The drawing under review shows one solid part. Ordinate dimensions are in mm from its lowest x, y, z. A direction names the side the tool comes from. Round coordinates to 2 decimals unless told otherwise and drop trailing zeros. Order: outer loops, then holes, each group sorted by start corner. A loop starts at its lowest first (then second) coordinate and runs counter-clockwise, first axis right, second up. Notation, with made-up numbers: M 80.5,75.25 L 111.5,75.25 A15 ccw 111.5,95.25 Z; hole C 84.5,46.25 d3. An arc over 180 degrees is marked long. Answer as a JSON object with one key per item and string values. Group by question number.
1) The part is to be moulded in two halves that separate along X. For the marked faces 1, 2, 3 and 4, say which applies: +X half, -X half, draft (parallel to the pull), parting line (faces both ways), or undercut.
2) Consider section B-B, the plane y = 14.5. Write out the cut boundary in (x, z).
3) For the marked faces 5, 6 and 7, list the 3-axis set-ups (+Z, -Z, +X, -X, +Y, -Y) from which the entire face can be reached by the end or side of a thin tool; tool diameter is ignored.
4) To check wall thickness, follow line 1 (X direction, y = 10.75, z = 70.5); line 2 (X direction, y = 3, z = 18); line 3 (X direction, y = 15.75, z = 56). State the ranges of each line that lie inside material, in increasing order.
5) Consider section C-C, the plane z = 5. Write out the cut boundary in (x, y).
6) Consider section A-A, the plane z = 76. Write out the cut boundary in (x, y), then the cut area to 3 significant figures.
7) Insertion check: pin 1 Ø2.5 at (y, z) = (8, 40.5) entering from +X; pin 2 Ø0.8 at (x, y) = (57, 8) entering from -Z; pin 3 Ø10 at (y, z) = (4.5, 9.5) entering from +X. Each pin has a flat end and moves straight along its axis. Give the tip position at first contact, or say it passes through.
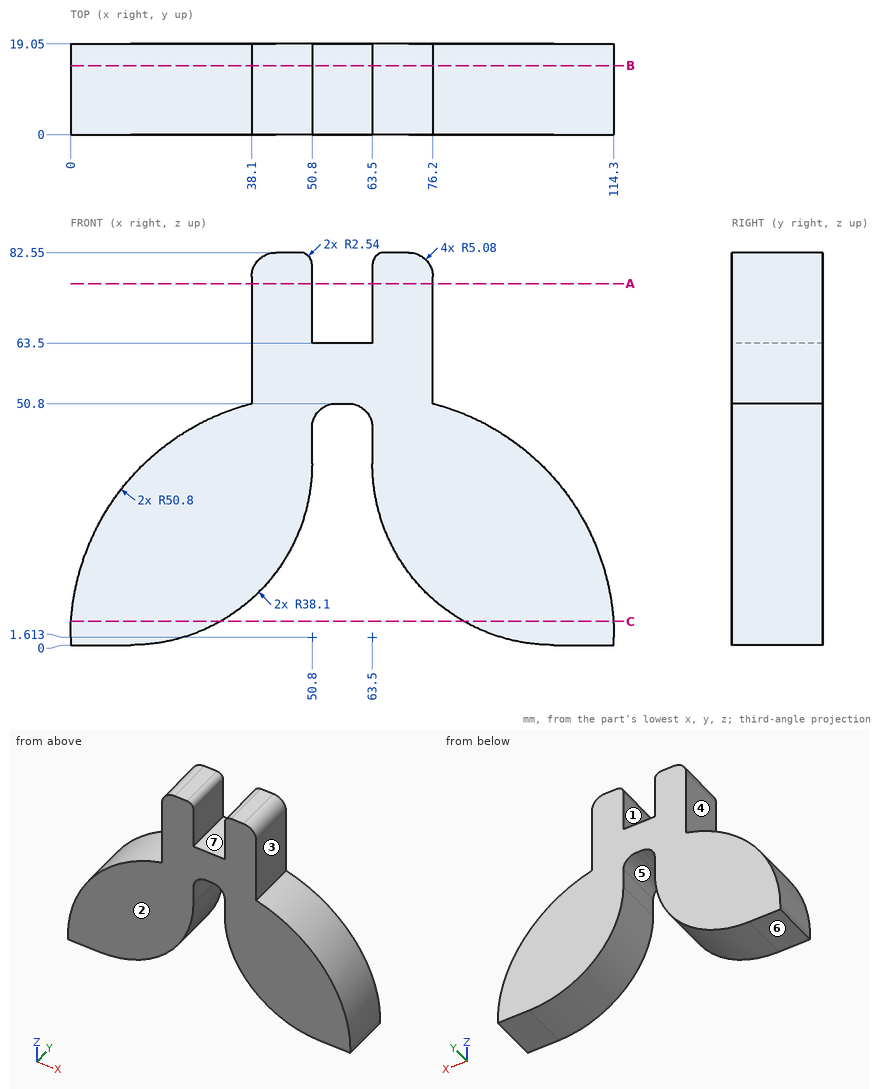
Results list:
{
 "1": {"face 1": "undercut", "face 2": "draft", "face 3": "+X half", "face 4": "-X half"},
 "2": {"outline": "M 0,0 L 12.7,0 A38.1 ccw 50.8,38.1 L 50.8,45.72 A5.08 cw 55.88,50.8 L 58.42,50.8 A5.08 cw 63.5,45.72 L 63.5,38.1 A38.1 ccw 101.6,0 L 114.3,0 L 114.3,1.61 A50.8 ccw 76.2,50.8 L 76.2,77.47 A5.08 ccw 71.12,82.55 L 66.04,82.55 A2.54 ccw 63.5,80.01 L 63.5,63.5 L 50.8,63.5 L 50.8,80.01 A2.54 ccw 48.26,82.55 L 43.18,82.55 A5.08 ccw 38.1,77.47 L 38.1,50.8 A50.8 ccw 0,1.61 Z"},
 "3": {"face 5": "-Z, +Y, -Y", "face 6": "-Z, +X, -X, +Y, -Y", "face 7": "+Z, +Y, -Y"},
 "4": {"line 1": "38.1 to 50.8, 63.5 to 76.2", "line 2": "2.72 to 45.07, 69.23 to 111.58", "line 3": "38.1 to 76.2"},
 "5": {"outline": "M 0.11,0 L 31.57,0 L 31.57,19.05 L 0.11,19.05 Z; M 82.73,0 L 114.19,0 L 114.19,19.05 L 82.73,19.05 Z"},
 "6": {"outline": "M 38.1,0 L 50.8,0 L 50.8,19.05 L 38.1,19.05 Z; M 63.5,0 L 76.2,0 L 76.2,19.05 L 63.5,19.05 Z", "area": "484 mm^2"},
 "7": {"pin 1": "x = 97.62", "pin 2": "z = 50.8", "pin 3": "x = 114.22"}
}
